Answer from the drawing. Dimensions are ordinates in mm from the lowest x, y and z of the part. A direction names the side the tool comes from. Give positions to 0.01 mm unless a question says otherwise; leave off trailing zeros. Order: outer loops, then holes, each group sorted by start corner. A loop starts at its lowest first (then second) coordinate and runs counter-clockwise, first axis right, second up. Notation, with made-up numbers: (52.5, 56) - (70.5, 56) arc R27 ccw to (70.5, 84) - close; hole circle Ø8 at (-29.5, 62). An arc over 180 degrees is marked (long way). Answer in a Markdown table with one row per item.
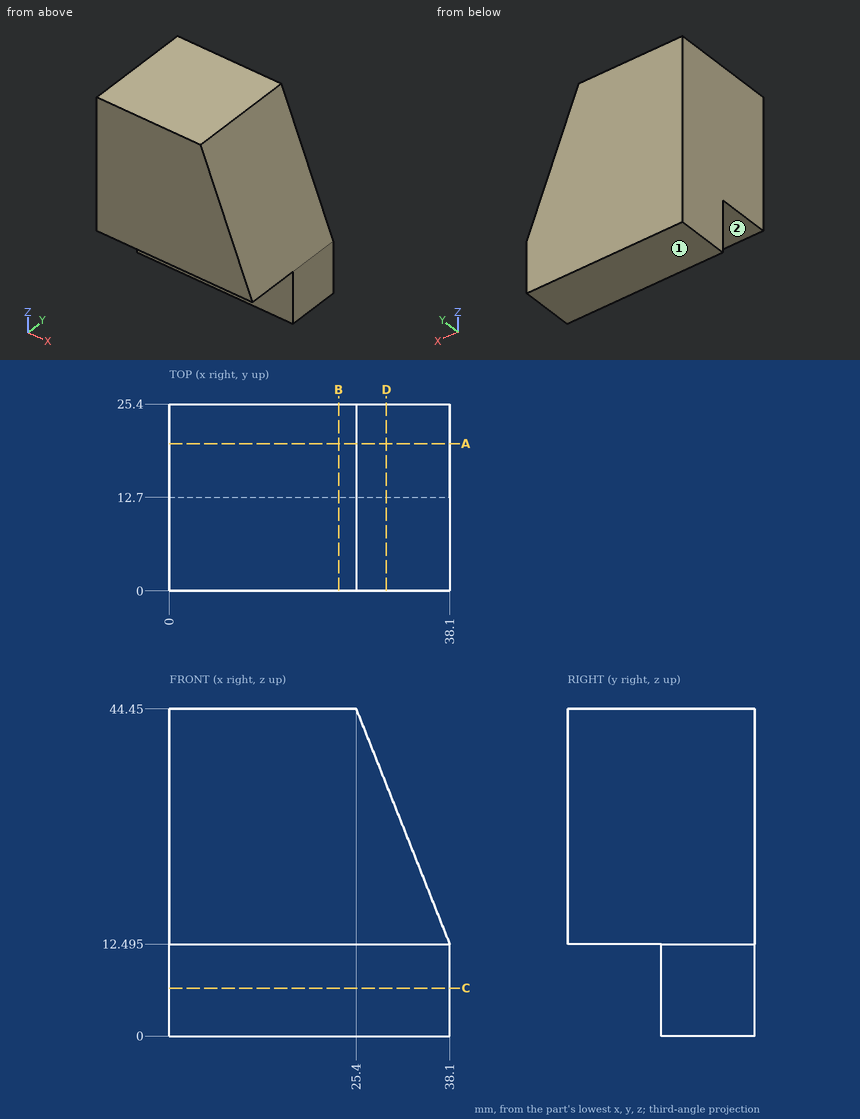
Item 1: Consider line 1 (Z direction, x = 3.5, y = 9.75) (3 decimals); line 2 (Y direction, x = 4, z = 7.5); line 3 (X direction, y = 13.5, z = 28). Determine where each line is inside the solid, lowest interval first.
Answer block:
| item | result |
|---|---|
| line 1 | 12.495 to 44.45 |
| line 2 | 12.7 to 25.4 |
| line 3 | 0 to 31.94 |
Item 2: Find section C-C on z = 6.5. Write down the section's boundary in (x, y).
Answer block:
| item | result |
|---|---|
| outline | (0, 12.7) - (38.1, 12.7) - (38.1, 25.4) - (0, 25.4) - close |
Item 3: Which of the six approach directions +Z, -Z, +X, -X, +Y, -Y give full straight-line access (tool end or side, diameter ignored) to the marked faces 1 and 2?
Answer block:
| item | result |
|---|---|
| face 1 | -Z, +X, -X, +Y, -Y |
| face 2 | -Z, +X, -X, -Y |
Item 4: Each of these flat-tipped pins is pushed along its axis until it touches: P1, Ø10, axis at y = 12, z = 27.5, coming from the +X side; P2, Ø1.5, axis at x = 11.5, y = 6.5, coming from the -Z side (3 decimals); P3, Ø6, axis at x = 24, z = 9, coming from the -Y side. Where does it stop, or does it pass through?
Answer block:
| item | result |
|---|---|
| P1 | x = 34.12 |
| P2 | z = 12.495 |
| P3 | y = 12.7 |
Item 5: Find section B-B on x = 23. Write down the section's boundary in (y, z) (3 decimals).
Answer block:
| item | result |
|---|---|
| outline | (0, 12.495) - (12.7, 12.495) - (12.7, 0) - (25.4, 0) - (25.4, 44.45) - (0, 44.45) - close |
Item 6: Find section D-D on x = 29.5. Write down the section's boundary in (y, z) (3 decimals), then the cut area to 3 significant figures.
Answer block:
| item | result |
|---|---|
| outline | (0, 12.495) - (12.7, 12.495) - (12.7, 0) - (25.4, 0) - (25.4, 34.134) - (0, 34.134) - close |
| area | 708 mm² |
Item 7: Find section A-A on y = 20. Write down the section's boundary in (x, z) (3 decimals), then the cut area to 3 significant figures.
Answer block:
| item | result |
|---|---|
| outline | (0, 0) - (38.1, 0) - (38.1, 12.495) - (25.4, 44.45) - (0, 44.45) - close |
| area | 1,490 mm² |
